Here's how the part is built. I have some questions about the finished solid (model axes, mm). A direction names the side the tool comes from. Coordinates: 2 decimals unless noted, no trailing zeros. Order: outer loops, then holes, each group sorted by start corner. A loop starts at its lowest first (then second) coordinate and runs counter-clockwise, first axis right, second up. Notation, with made-up numbers: (68.5, 83.5) - (118.5, 83.5) arc R17 ccw to (118.5, 113.5) - close; hole circle Ø4 at (-15.75, -7). An arc over 180 degrees is marked (long way). Answer as CSV lines item,"result". Start each with the question number.
Q1. Thinking about a two-plate mould opening in X: for faces 1 (the face through (0, 5.51, 8)), 2 (the face through (0, 9, 2)), 3 (the face through (0, 5.5, 0)), 4 (the face through (-3.75, -3, -9)), which applies, released by +X, released by -X, zero draft, split by the parting line, or undercut?
Q2. Suppose I cut it at C-C (y = 0). Please give me the cut outline in (x, z), then the cut area to 3 significant figures.
Q3. I need wall thicknesses on line 1 (X direction, y = 11.75, z = 0); line 2 (Z direction, x = 6.25, y = 0.5); line 3 (X direction, y = -3.25, z = -0.75). Which ranges of each line are inside material? Lowest first, please.
Q4. For pin 1 Ø2 at (x, z) = (-3, 3.5) entering from +Y; pin 2 Ø3 at (y, z) = (8, -5) entering from +X; pin 3 Ø0.8 at (y, z) = (-6.5, 5) entering from -X; pin 4 Ø8 at (y, z) = (10, -4) entering from +X, each with a flat end and sliding along its axis, tell me the tip position at first contact or that it passes through.
Q5. Suppose I cut it at D-D (x = -5.5). Please give me the cut outline in (y, z).
Q6. Suppose I cut it at A-A (y = 6.25). Please give me the cut outline in (x, z), then the cut area to 3 significant figures.
Q7. For faces 5 (the face through (-8, -1, 4.75)), 6 (the face through (-6.2, -7, -5)), 7 (the face through (7, -2.5, 0)), which set-ups out of +Z, -Z, +X, -X, +Y, -Y let a thin tool reach every point of the face, with its end or its side?
from build123d import *

# Parameters (mm, degrees)
SKETCH2_W           = 13
SKETCH2_H           = 11
BOSS_EXTRUDE1_DEPTH = 6.5
BOSS_EXTRUDE2_DEPTH = 1
SKETCH4_W           = 9.5
SKETCH4_H           = 11
BOSS_EXTRUDE3_DEPTH = 3
CHAMFER1_SIZE       = 2
SKETCH5_W           = 9.5
SKETCH5_H           = 11
BOSS_EXTRUDE4_DEPTH = 3
CHAMFER2_SIZE       = 2
SKETCH6_W           = 9
SKETCH6_H           = 1.5
BOSS_EXTRUDE5_DEPTH = 5
SKETCH7_W           = 7.5
SKETCH7_H           = 3
BOSS_EXTRUDE6_DEPTH = 4.5
SKETCH8_R           = 0.5
BOSS_EXTRUDE7_DEPTH = 8
FILLET2_R           = 0.25
SKETCH9_W           = 3
SKETCH9_H           = 5.5
SKETCH9_W_2         = 5.5
SKETCH9_H_2         = 3
BOSS_EXTRUDE8_DEPTH = 0.01
SKETCH10_W          = 0.3
SKETCH10_H          = 1
SKETCH10_W_2        = 0.1
SKETCH10_H_2        = 0.75
SKETCH10_W_3        = 0.75
SKETCH10_H_3        = 0.1
SKETCH10_W_4        = 0.25
SKETCH10_H_4        = 0.25
BOSS_EXTRUDE9_DEPTH = 3
CHAMFER3_SIZE       = 0.25
CHAMFER4_SIZE       = 0.1


with BuildPart() as part:
    # Sketch2 → Boss-Extrude1 (new, symmetric)
    with BuildSketch(Plane(origin=(0, 0, 0), x_dir=(0, 0, -1), z_dir=(1, 0, 0))):
        Rectangle(SKETCH2_W, SKETCH2_H)
    extrude(amount=BOSS_EXTRUDE1_DEPTH, both=True)

    # Sketch3 → Boss-Extrude2 (add)
    with BuildSketch(Plane(origin=(6.5, 0, 0), x_dir=(0, 0, -1), z_dir=(1, 0, 0))):
        Polygon((3, -1.5), (-3, -1.5), (-3, -5.5), (-2, -5.5), (-2, -2.5), (2, -2.5), (2, -5.5), (3, -5.5), align=None)
    extrude(amount=BOSS_EXTRUDE2_DEPTH)

    # Sketch4 → Boss-Extrude3 (add)
    with BuildSketch(Plane.XY.offset(6.5)):
        Rectangle(SKETCH4_W, SKETCH4_H)
    extrude(amount=BOSS_EXTRUDE3_DEPTH)

    # Chamfer1
    chamfer1_edges = [part.edges().sort_by_distance(p)[0] for p in [
        (-4.75, 5.5, 8),
        (4.75, 5.5, 8),
    ]]
    chamfer(chamfer1_edges, length=CHAMFER1_SIZE)

    # Sketch5 → Boss-Extrude4 (add)
    with BuildSketch(Plane.ZY.offset(6.5)):
        Rectangle(SKETCH5_W, SKETCH5_H)
    extrude(amount=BOSS_EXTRUDE4_DEPTH)

    # Chamfer2
    chamfer2_edges = [part.edges().sort_by_distance(p)[0] for p in [
        (-8, 5.5, -4.75),
        (-8, 5.5, 4.75),
    ]]
    chamfer(chamfer2_edges, length=CHAMFER2_SIZE)

    # Sketch6 → Boss-Extrude5 (add)
    with BuildSketch(Plane(origin=(0, 0, -6.5), x_dir=(-1, 0, 0), z_dir=(0, 0, -1))):
        with Locations((0, -4.75)):
            Rectangle(SKETCH6_W, SKETCH6_H)
    extrude(amount=BOSS_EXTRUDE5_DEPTH)

    # Sketch7 → Boss-Extrude6 (add)
    with BuildSketch(Plane(origin=(0, 0, -6.5), x_dir=(-1, 0, 0), z_dir=(0, 0, -1))):
        with Locations((0, -2.5)):
            Rectangle(SKETCH7_W, SKETCH7_H)
    extrude(amount=BOSS_EXTRUDE6_DEPTH)

    # Sketch8 → Boss-Extrude7 (add)
    with BuildSketch(Plane(origin=(0, 5.5, 0), x_dir=(1, 0, 0), z_dir=(0, 1, 0))):
        with BuildLine():
            Line((1.5, 0.5), (1.5, -0.5))
            ThreePointArc((1.5, -0.5), (0, -2), (-1.5, -0.5))
            Line((-1.5, -0.5), (-1.5, 0.5))
            ThreePointArc((-1.5, 0.5), (0, 2), (1.5, 0.5))
        make_face()
        with Locations(Location((0, 0, 0), (0, 0, 270))):
            Circle(SKETCH8_R, mode=Mode.SUBTRACT)
    extrude(amount=BOSS_EXTRUDE7_DEPTH)

    # Fillet2
    fillet2_edges = [part.edges().sort_by_distance(p)[0] for p in [
        (0, 13.5, -2),
        (-1.5, 13.5, 0),
        (0, 13.5, 2),
        (1.5, 13.5, 0),
        (0, 13.5, -0.5),
    ]]
    fillet(fillet2_edges, radius=FILLET2_R)

    # Sketch9 → Boss-Extrude8 (add)
    with BuildSketch(Plane(origin=(0, 5.5, 0), x_dir=(1, 0, 0), z_dir=(0, 1, 0))):
        with Locations((-8, 0)):
            Rectangle(SKETCH9_W, SKETCH9_H)
        with Locations((0, -8)):
            Rectangle(SKETCH9_W_2, SKETCH9_H_2)
    extrude(amount=BOSS_EXTRUDE8_DEPTH)

    # Sketch10 → Boss-Extrude9 (add)
    with BuildSketch(Plane.XZ.offset(5.5)):
        with Locations((-6.35, -5)):
            Rectangle(SKETCH10_W, SKETCH10_H)
        with Locations((6.35, -5)):
            Rectangle(SKETCH10_W, SKETCH10_H)
        with Locations((-6.35, 5)):
            Rectangle(SKETCH10_W, SKETCH10_H)
        with Locations((6.35, 5)):
            Rectangle(SKETCH10_W, SKETCH10_H)
        with Locations((-9.15, 0)):
            Rectangle(SKETCH10_W_2, SKETCH10_H_2)
        with Locations((-9.15, -2.5)):
            Rectangle(SKETCH10_W_2, SKETCH10_H_2)
        with Locations((-9.15, 2.5)):
            Rectangle(SKETCH10_W_2, SKETCH10_H_2)
        with Locations((0, 9)):
            Rectangle(SKETCH10_W_3, SKETCH10_H_3)
        with Locations((-2.5, 9)):
            Rectangle(SKETCH10_W_3, SKETCH10_H_3)
        with Locations((2.5, 9)):
            Rectangle(SKETCH10_W_3, SKETCH10_H_3)
        with Locations((-3.1, -5.5)):
            Rectangle(SKETCH10_W_4, SKETCH10_H_4)
        with Locations((2.9, -5.5)):
            Rectangle(SKETCH10_W_4, SKETCH10_H_4)
        with Locations((2.9, -9.5)):
            Rectangle(SKETCH10_W_4, SKETCH10_H_4)
        with Locations((-3.1, -9.5)):
            Rectangle(SKETCH10_W_4, SKETCH10_H_4)
    extrude(amount=BOSS_EXTRUDE9_DEPTH)

    # Chamfer3
    chamfer3_edges = [part.edges().sort_by_distance(p)[0] for p in [
        (-6.35, -8.5, -5.5),
        (-6.35, -8.5, -4.5),
        (6.35, -8.5, -4.5),
        (6.35, -8.5, -5.5),
        (-6.35, -8.5, 4.5),
        (-6.35, -8.5, 5.5),
        (6.35, -8.5, 5.5),
        (6.35, -8.5, 4.5),
        (-9.15, -8.5, 0.375),
        (-9.15, -8.5, -0.375),
        (-9.15, -8.5, -2.125),
        (-9.15, -8.5, -2.875),
        (-9.15, -8.5, 2.875),
        (-9.15, -8.5, 2.125),
        (0.375, -8.5, 9),
        (-0.375, -8.5, 9),
        (-2.125, -8.5, 9),
        (-2.875, -8.5, 9),
        (2.875, -8.5, 9),
        (2.125, -8.5, 9),
    ]]
    chamfer(chamfer3_edges, length=CHAMFER3_SIZE)

    # Chamfer4
    chamfer4_edges = [part.edges().sort_by_distance(p)[0] for p in [
        (3.025, -8.5, -5.5),
        (2.9, -8.5, -5.375),
        (2.775, -8.5, -5.5),
        (2.9, -8.5, -5.625),
        (-2.975, -8.5, -5.5),
        (-3.1, -8.5, -5.375),
        (-3.225, -8.5, -5.5),
        (-3.1, -8.5, -5.625),
        (3.025, -8.5, -9.5),
        (2.9, -8.5, -9.375),
        (2.775, -8.5, -9.5),
        (2.9, -8.5, -9.625),
        (-2.975, -8.5, -9.5),
        (-3.1, -8.5, -9.375),
        (-3.225, -8.5, -9.5),
        (-3.1, -8.5, -9.625),
    ]]
    chamfer(chamfer4_edges, length=CHAMFER4_SIZE)


solid = part.part
Here are the results:
1,face 1,"zero draft"
1,face 2,"split by the parting line"
1,face 3,"undercut"
1,face 4,"released by -X"
2,outline,"(-9.5, -4.75) - (-6.5, -4.75) - (-6.5, -6.5) - (6.5, -6.5) - (6.5, 6.5) - (4.75, 6.5) - (4.75, 9.5) - (-4.75, 9.5) - (-4.75, 6.5) - (-6.5, 6.5) - (-6.5, 4.75) - (-9.5, 4.75) - close"
2,area,"226 mm²"
3,line 1,"x = -1.5 to -0.5, 0.5 to 1.5"
3,line 2,"z = -6.5 to 6.5"
3,line 3,"x = -9.5 to 6.5"
4,pin 1,"stops at y = 5.5"
4,pin 2,"passes through"
4,pin 3,"stops at x = -6.5"
4,pin 4,"stops at x = 1.5"
5,outline,"(-5.5, -6.5) - (5.5, -6.5) - (5.5, 6.5) - (-5.5, 6.5) - close"
6,outline,"(-1.5, -0.5) arc R1.5 ccw to (1.5, -0.5) - (1.5, 0.5) arc R1.5 ccw to (-1.5, 0.5) - close; hole circle Ø1 at (0, 0)"
6,area,"9.28 mm²"
7,face 5,"+Z, -X, +Y, -Y"
7,face 6,"+Z, -Z, -Y"
7,face 7,"+X, -Y"
